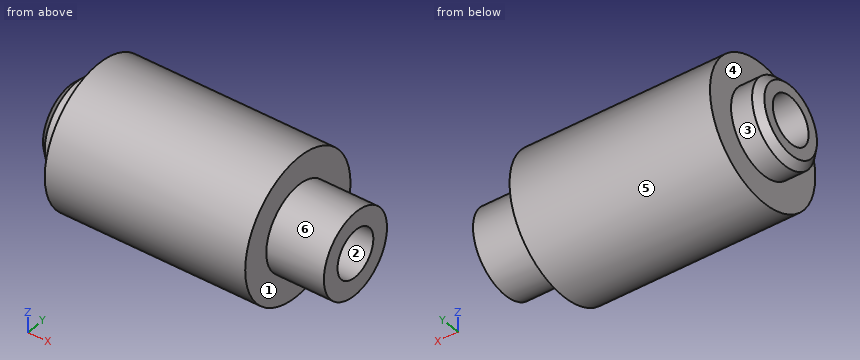
```python
from build123d import *

# Parameters (mm, degrees)
ESQUISSE1_R        = 5
BOSS_EXTRU_1_DEPTH = 14.275
ESQUISSE5_R        = 3
BOSS_EXTRU_2_DEPTH = 2
CHANFREIN1_SIZE    = 0.5
BOSS_EXTRU_3_START = 4.1
ESQUISSE6_R        = 3
BOSS_EXTRU_3_DEPTH = 4.1
D_GAGEMENT_M32_D   = 3.4


with BuildPart() as part:
    # Esquisse1 → Boss.-Extru.1 (new body)
    with BuildSketch(Plane(origin=(0, 0, 0), x_dir=(0, 0, -1), z_dir=(1, 0, 0))):
        Circle(ESQUISSE1_R)
    extrude(amount=BOSS_EXTRU_1_DEPTH)

    # Esquisse5 → Boss.-Extru.2 (add)
    with BuildSketch(Plane.ZY):
        Circle(ESQUISSE5_R)
    extrude(amount=BOSS_EXTRU_2_DEPTH)

    # Chanfrein1
    chanfrein1_edges = [part.edges().sort_by_distance(p)[0] for p in [
        (-2, 0, -3),
    ]]
    chamfer(chanfrein1_edges, length=CHANFREIN1_SIZE)

    # Esquisse6 → Boss.-Extru.3 (add)
    with BuildSketch(Plane(origin=(14.275, 0, 0), x_dir=(0, 0, -1), z_dir=(1, 0, 0)).offset(BOSS_EXTRU_3_START)):
        with Locations(Location((0, 0, 0), (0, 0, 180))):
            Circle(ESQUISSE6_R)
    extrude(amount=-BOSS_EXTRU_3_DEPTH)

    # Dégagement M32 (through all)
    with Locations(Plane(origin=(18.375, 0, 0), x_dir=(0, 0, -1), z_dir=(1, 0, 0))):
        with Locations((0, 0)):
            Hole(D_GAGEMENT_M32_D / 2)


solid = part.part
```
Verification items for the finished model (mm, model axes). Face numbers are marked on the shaded views. A direction names the side the tool comes from. Round coordinates to 2 decimals unless told otherwise and drop trailing zeros. Write each loop counter-clockwise with the first axis right and the second up, starting at its lowest first coordinate (ties: lowest second). Pieces come first, ordered by that corner, then holes. Notation, with made-up numbers: (33, 53.25) -> (78, 53.25) arc R23 cw to (78, 68.25) -> close; hole circle Ø10 at (0.25, 36.25). An arc over 180 degrees is marked (long way). Write each question's results on one line, items separated by ' | '. Start each with the question number.
1. Cross-section at A-A (z = 0). Enter the section's corners in (x, y) (3 decimals), then the cut area to 3 significant figures.
2. Cross-section at D-D (x = 6.75). Enter the section's corners in (y, z), then the cut area to 3 significant figures.
3. Set-up check for the marked faces 4, 5 and 6: record each of +Z, -Z, +X, -X, +Y, -Y from which the full face is reachable in a straight line by a thin tool's end or side.
4. Depth check by flat-ended pin: P1, Ø3, axis at x = 5, z = -2.5, coming from the -Y side; P2, Ø1.5, axis at y = -3.5, z = 2.5, coming from the -X side. Enter the tip coordinate at first touch or a pass-through.
5. Material ranges on probe 1 along Y at (x, z) = (2.75, 0); probe 2 along Y at (x, z) = (12.25, -4); probe 3 along Y at (x, z) = (6.75, 1), recorded low to high. Write a range as from..to.
6. Cross-section at C-C (x = 15). Enter the section's corners in (y, z), then the cut area to 3 significant figures.
7. Draft check along Y on the marked faces 1, 2 and 3. Enter one of: +Y half, -Y half, draft (parallel to the pull), parting line (faces both ways), or undercut.
Solutions:
1) outline: (-2, -2.5) -> (-1.5, -3) -> (0, -3) -> (0, -5) -> (14.275, -5) -> (14.275, -3) -> (18.375, -3) -> (18.375, -1.7) -> (-2, -1.7) -> close; (-2, 1.7) -> (18.375, 1.7) -> (18.375, 3) -> (14.275, 3) -> (14.275, 5) -> (0, 5) -> (0, 3) -> (-1.5, 3) -> (-2, 2.5) -> close | area: 110 mm2
2) outline: circle Ø10 at (0, 0); hole circle Ø3.4 at (0, 0) | area: 69.5 mm2
3) face 4: -X | face 5: +X, -X | face 6: +X
4) P1: stops at y = -4.9 | P2: stops at x = 0
5) probe 1: y = -5..-1.7, 1.7..5 | probe 2: y = -3..3 | probe 3: y = -4.9..-1.37, 1.37..4.9
6) outline: circle Ø6 at (0, 0); hole circle Ø3.4 at (0, 0) | area: 19.2 mm2
7) face 1: draft | face 2: undercut | face 3: parting line
